Input: part model. Units: mm. Frame: model coordinates. Face numbers are marked on the shaded views. A direction names the side the tool comes from. Give positions to 0.01 mm unless a question says otherwise; leave off trailing zeros. Loops run counter-clockwise (first coordinate to the right, second up) from the corner with the lowest first, then second, coordinate; pieces in that order, holes last. Notation, with made-up numbers: M 7.5,31.5 L 32.5,31.5 A19 ccw 32.5,53.5 Z; hole C 85.5,-12 d3. An arc over 180 degrees is marked long. Answer as a JSON object with one key per item and string values. Group by question number.
```python
from build123d import *

# Parameters (mm, degrees)
Y_KSEKLIK_EKSTR_ZYON1_DEPTH = 6.5
IZIM2_R                     = 5
Y_KSEKLIK_EKSTR_ZYON2_DEPTH = 120
RADYUS1_R                   = 0.5


with BuildPart() as part:
    # Çizim1 → Yükseklik-Ekstrüzyon1 (new body)
    with BuildSketch(Plane.XY):
        Polygon((9.814954576, 0), (4.907477288, 8.5), (-4.907477288, 8.5), (-9.814954576, 0), (-4.907477288, -8.5), (4.907477288, -8.5), align=None)
    extrude(amount=Y_KSEKLIK_EKSTR_ZYON1_DEPTH)

    # Çizim2 → Yükseklik-Ekstrüzyon2 (add)
    with BuildSketch(Plane.XY.offset(6.5)):
        Circle(IZIM2_R)
    extrude(amount=Y_KSEKLIK_EKSTR_ZYON2_DEPTH)

    # Çizim3 → Kes-Döndür1 (revolve, cut)
    with BuildSketch(Plane(origin=(0, 0, 0), x_dir=(1, 0, 0), z_dir=(0, 1, 0))):
        Polygon((-9.814954576, 0), (-8.814954576, 0), (-9.814954576, -0.5), align=None)
        Polygon((-9.814954576, -6.5), (-9.814954576, -6), (-8.814954576, -6.5), align=None)
    revolve(axis=Axis((0, 0, 0), (0, 0, 1)), mode=Mode.SUBTRACT)

    # Radyus1
    radyus1_edges = [part.edges().sort_by_distance(p)[0] for p in [
        (-5, 0, 126.5),
    ]]
    fillet(radyus1_edges, radius=RADYUS1_R)


solid = part.part
```
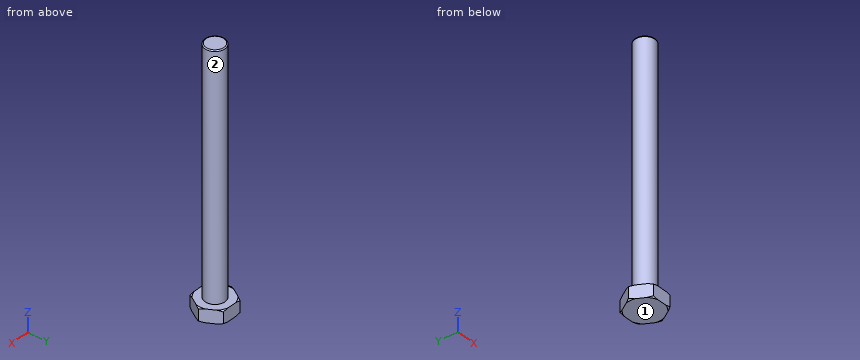
1. Reachability of the marked faces 1 and 2 from +Z, -Z, +X, -X, +Y, -Y: full face, straight path, thin tool, end or side. Return the list, or none.
2. First-contact query: P1, Ø1.5, axis at x = -5, y = 6.5, coming from the -Z side; P2, Ø3, axis at x = 7, y = -5, coming from the +Z side; P3, Ø6, axis at y = 6.5, z = 31.5, coming from the +X side; P4, Ø3, axis at x = 7.5, z = 76, coming from the -Y side. Flat tips, straight axial feed; report the tip coordinate or a pass-through.
3. Section B-B (z = 56). Output: boundary loops of the cut face in (x, y).
4. Material intervals for L1, parallel to Z at x = -5.25, y = 4.25; L2, parallel to Z at x = 3.5, y = 3; L3, parallel to Y at x = -3.75, z = 56.5, sorted ascending.
5. Section A-A (x = 0). Output: boundary loops of the cut face in (y, z), then the cut area to 3 significant figures.
Geometry results:
{
 "1": {"face 1": "-Z, +X, -X, +Y, -Y", "face 2": "+Z"},
 "2": {"P1": "z = 0", "P2": "z = 6.5", "P3": "x = 3.57", "P4": "through"},
 "3": {"outline": "C 0,0 d10"},
 "4": {"L1": "0 to 6.5", "L2": "0 to 126.49", "L3": "-3.31 to 3.31"},
 "5": {"outline": "M -8.5,0 L 8.5,0 L 8.5,6.5 L 5,6.5 L 5,126 A0.5 ccw 4.5,126.5 L -4.5,126.5 A0.5 ccw -5,126 L -5,6.5 L -8.5,6.5 Z", "area": "1,310 mm2"}
}
